from build123d import *

# Parameters (mm, degrees)
SKETCH_1_R          = 2
SKETCH_1_W          = 3
SKETCH_1_H          = 50
SKETCH_1_R_2        = 70
SKETCH_1_R_3        = 22.5
EXTRUDE_1_DEPTH     = 5
SKETCH_2_R          = 2
CUT_EXTRUDE_1_DEPTH = 697.437362582
SKETCH_3_R          = 1.5
CUT_EXTRUDE_2_DEPTH = 697.437362582
SKETCH_4_R          = 2
CUT_EXTRUDE_3_DEPTH = 10


with BuildPart() as part:
    # 草图1 → 凸台-拉伸1 (new body)
    # profile 1 of 2: a face of its own
    with BuildSketch(Plane.XY):
        with BuildLine():
            ThreePointArc((-184.975195398, 573.957266214), (-108.724882678, 291.977251427), (-100, 0))
            Line((-100, 0), (-100, -10))
            Line((-100, -10), (-91, -10))
            Line((-91, -10), (-91, 11))
            Line((-91, 11), (-69, 11))
            Line((-69, 11), (-69, -10))
            Line((-69, -10), (100, -10))
            Line((100, -10), (100, 0))
            ThreePointArc((100, 0), (62.740102222, 327.663103245), (-58.911784918, 634.179379428))
            ThreePointArc((-58.911784918, 634.179379428), (-52.264577008, 617.661043914), (-50, 600))
            ThreePointArc((-50, 600), (-106.738470636, 531.267679808), (-184.975195398, 573.957266214))
        make_face()
        with Locations((-50, 0)):
            Circle(SKETCH_1_R, mode=Mode.SUBTRACT)
        Circle(SKETCH_1_R, mode=Mode.SUBTRACT)
        with Locations((50, 0)):
            Circle(SKETCH_1_R, mode=Mode.SUBTRACT)
        with Locations((-91.5, 435)):
            Rectangle(SKETCH_1_W, SKETCH_1_H, mode=Mode.SUBTRACT)
        with Locations((-68.5, 435)):
            Rectangle(SKETCH_1_W, SKETCH_1_H, mode=Mode.SUBTRACT)
    # profile 2 of 2: a face of its own
    with BuildSketch(Plane.XY):
        with Locations((-120, 600)):
            Circle(SKETCH_1_R_2)
        with Locations((-120, 600)):
            Circle(SKETCH_1_R_3, mode=Mode.SUBTRACT)
    extrude(amount=EXTRUDE_1_DEPTH)

    # 草图2 → 切除-拉伸1 (cut, through all)
    with BuildSketch(Plane(origin=(0, 0, 0), x_dir=(-1, 0, 0), z_dir=(0, 0, -1))):
        with Locations((80, 386.410161514)):
            Circle(SKETCH_2_R)
        with Locations((80, 371.410161514)):
            Circle(SKETCH_2_R)
        with Locations((80, 356.410161514)):
            Circle(SKETCH_2_R)
        with Locations((56.339745962, 352.749907476)):
            Circle(SKETCH_2_R)
        with Locations((46.339745962, 335.4293994)):
            Circle(SKETCH_2_R)
        with Locations((26.339745962, 300.788383249)):
            Circle(SKETCH_2_R)
        with Locations((6.339745962, 266.147367097)):
            Circle(SKETCH_2_R)
        with Locations((-13.660254038, 231.506350946)):
            Circle(SKETCH_2_R)
        with Locations((80, 76.410161514)):
            Circle(SKETCH_2_R)
        with Locations((80, 116.410161514)):
            Circle(SKETCH_2_R)
        with Locations((80, 236.410161514)):
            Circle(SKETCH_2_R)
        with Locations((80, 276.410161514)):
            Circle(SKETCH_2_R)
        with Locations((80, 316.410161514)):
            Circle(SKETCH_2_R)
    extrude(amount=-CUT_EXTRUDE_1_DEPTH, mode=Mode.SUBTRACT)

    # 草图3 → 切除-拉伸2 (cut, through all)
    with BuildSketch(Plane.XY.offset(5)):
        with Locations((-120, 636.5)):
            Circle(SKETCH_3_R)
        with Locations((-96.538252246, 627.960622174)):
            Circle(SKETCH_3_R)
        with Locations((-84.054517015, 606.338158485)):
            Circle(SKETCH_3_R)
        with Locations((-88.390072762, 581.75)):
            Circle(SKETCH_3_R)
        with Locations((-107.516264769, 565.701219341)):
            Circle(SKETCH_3_R)
        with Locations((-132.483735231, 565.701219341)):
            Circle(SKETCH_3_R)
        with Locations((-151.609927238, 581.75)):
            Circle(SKETCH_3_R)
        with Locations((-155.945482985, 606.338158485)):
            Circle(SKETCH_3_R)
        with Locations((-143.461747754, 627.960622174)):
            Circle(SKETCH_3_R)
    extrude(amount=-CUT_EXTRUDE_2_DEPTH, mode=Mode.SUBTRACT)


with BuildPart() as body_2:
    # Split Bodies 1: the piece on the far side of the plane
    add(part.part)
    split(bisect_by=Plane(origin=(0, 325, 0), x_dir=(0, 0, -1), z_dir=(0, -1, 0)), keep=Keep.BOTTOM)

    # 草图4 → 切除-拉伸3 (cut)
    with BuildSketch(Plane.XY.offset(5)):
        with Locations((-21.595687559, 455)):
            Circle(SKETCH_4_R)
        with BuildLine():
            Line((-11.595687559, 325), (-11.595687559, 540.604962521))
            ThreePointArc((-11.595687559, 540.604962521), (30.836385122, 434.518144234), (63.404312441, 325))
            Line((63.404312441, 325), (-11.595687559, 325))
        make_face()
    extrude(amount=-CUT_EXTRUDE_3_DEPTH, mode=Mode.SUBTRACT)


with BuildPart() as part_1:
    add(part.part)

    # Split Bodies 1
    split(bisect_by=Plane(origin=(0, 325, 0), x_dir=(0, 0, -1), z_dir=(0, -1, 0)), keep=Keep.TOP)


solid = body_2.part
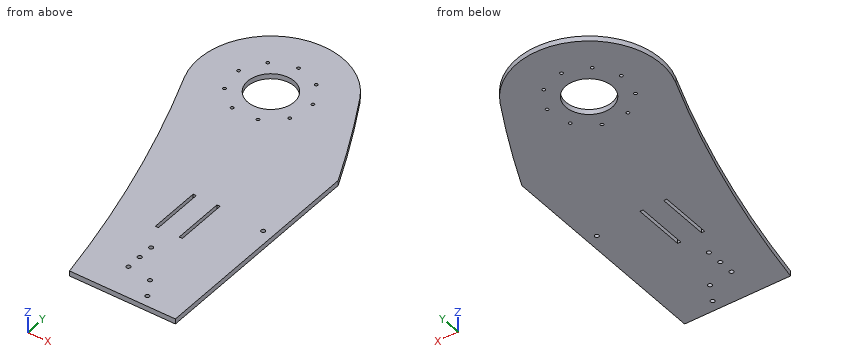
The listing builds one solid part. Answer for the finished solid, in the listing's coordinates (mm). Give positions to 0.01 mm unless a question says otherwise; leave off trailing zeros. Write each loop counter-clockwise with the first axis right and the second up, starting at its lowest first coordinate (ties: lowest second). Pieces come first, ordered by that corner, then holes. Notation, with made-up numbers: (48.25, -20) -> (89.25, -20) arc R17 cw to (89.25, -6) -> close; hole circle Ø10 at (50.25, -34). An arc over 180 degrees is marked (long way). Use a Markdown table: item, result.
(1) Find the intervals of material crossed by probe 1 along Y at (x, z) = (-81.5, 4.2); probe 2 along Y at (x, z) = (-80, 3.5); probe 3 along X at (y, z) = (439.5, 2.6), in increasing order. Write a range as from..to.
Return value:
| item | result |
|---|---|
| probe 1 | 325..355.09, 357.73..370.09, 372.73..385.09, 387.73..658.46 |
| probe 2 | 325..354.41, 358.41..369.41, 373.41..384.41, 388.41..657.45 |
| probe 3 | -139.76..-93, -90..-70, -67..-11.6 |
(2) Flat-ended cylindrical pins translate along their axes: P1, Ø1.5, axis at y = 603, z = 0.5, coming from the -X side; P2, Ø1.5, axis at x = -32, z = 3, coming from the +Y side. Find the tip coordinate at first contact, or state that the pin passes through.
Return value:
| item | result |
|---|---|
| P1 | x = -189.96 |
| P2 | y = 584.87 |
(3) Section C-C, the plane y = 463.5 is taken. Determine the outline of the cut face in (x, z), then the cut area to 3 significant figures.
Return value:
| item | result |
|---|---|
| outline | (-146.6, 0) -> (-11.6, 0) -> (-11.6, 5) -> (-146.6, 5) -> close |
| area | 675 mm2 |
(4) Section B-B, the plane y = 544 is taken. Determine the outline of the cut face in (x, z), then the cut area to 3 significant figures.
Return value:
| item | result |
|---|---|
| outline | (-173.41, 0) -> (-13.14, 0) -> (-13.14, 5) -> (-173.41, 5) -> close |
| area | 801 mm2 |
(5) Section A-A, the plane z = 3.75 is taken. Give the number of separate pieces and of enclosed holes in the cut face, then the cut area to 3 significant figures.
Return value:
| item | result |
|---|---|
| separate pieces | 1 |
| enclosed holes | 18 |
| area | 42,700 mm2 |
